Can you work these out from the drawing? Everything is in mm from the part's minimum corner. A direction names the side the tool comes from. Coordinates: 2 decimals unless noted, no trailing zeros. Loops run counter-clockwise (first coordinate to the right, second up) from the corner with the lowest first, then second, coordinate; pieces in that order, holes last. Notation, with made-up numbers: (77.25, 16) - (91.25, 16) arc R27 ccw to (91.25, 44) - close; hole circle Ø9 at (-6, 48). An arc over 180 degrees is marked (long way). Put each result on its own line as item: value. Start each with the question number.
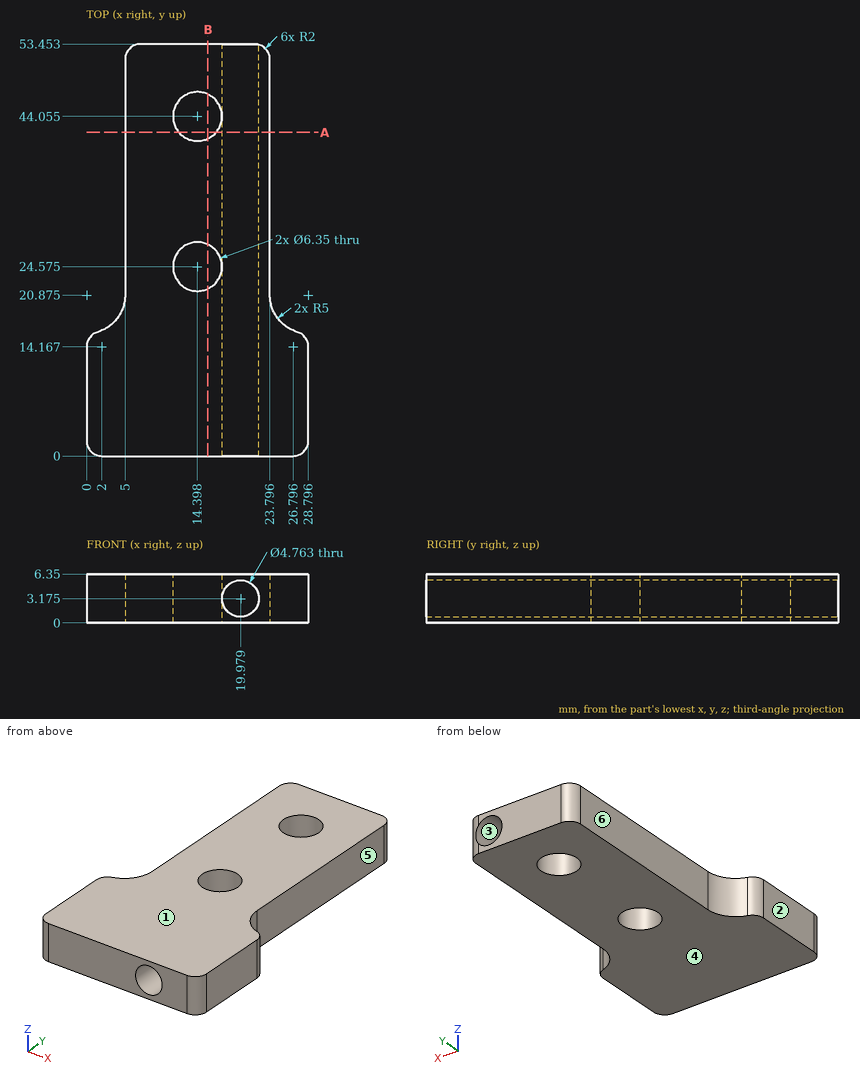
Q1. Will this pin go through, and if not, where does the flat tip stop? pin 1 (1.5 mm diameter, centred on x = 25, y = 35, fed in from -Z).
Q2. Please list where these lines run through material, in increasing order: line 1 along Y through (x, z) = (14.5, 1.5); line 2 along X through (y, z) = (23, 1.5) (1 decimal); line 3 along X through (y, z) = (26, 3.25) (1 decimal). Write a range as [from, to].
Q3. On a 3-axis mill with a long thin cutter (end or side, diameter ignored), from which of +Z, -Z, +X, -X, +Y, -Y can I reach the whole of each face in a straight line? I mean the marked faces 4, 5 and 6. Say none if no direction works.
Q4. I want a section at A-A on y = 42. Count the separate pieces of the cut face and the enclosed holes in it.
Q5. I want a section at B-B on x = 15.75. List the corners of the cut face in (y, z) for me.
Q6. We'd pull the mould along Z, two halves only. Please class the marked faces 1, 2 and 3: released by +Z, released by -Z, zero draft, split by the parting line, or undercut.
Calculated:
1. pin 1: through
2. line 1: [0, 21.4], [27.75, 40.88], [47.23, 53.45]
2. line 2: [5, 11.6], [17.2, 18.3], [21.7, 23.8]
2. line 3: [5, 11.6], [17.2, 17.6], [22.4, 23.8]
3. face 4: -Z, +X, -X, +Y, -Y
3. face 5: +Z, -Z, +X, +Y
3. face 6: +Z, -Z, -X, +Y
4. separate pieces: 2
4. enclosed holes: 1
5. outline: (0, 0) - (21.7, 0) - (21.7, 6.35) - (0, 6.35) - close; (27.45, 0) - (41.18, 0) - (41.18, 6.35) - (27.45, 6.35) - close; (46.93, 0) - (53.45, 0) - (53.45, 6.35) - (46.93, 6.35) - close
6. face 1: released by +Z
6. face 2: zero draft
6. face 3: undercut
